```python
from build123d import *

# Parameters (mm, degrees)
F0_R     = 3
F5_DEPTH = 25.501


with BuildPart() as f2:
    # F0 (on Front) → F2 (revolve)
    with BuildSketch(Plane.XZ):
        with BuildLine():
            ThreePointArc((-8, -6), (-15.455298, -3.701711), (-22.32268, 0))
            Line((-22.32268, 0), (-30, 0))
            Line((-30, 0), (-30, -32))
            ThreePointArc((-30, -32), (-22.5, -39.5), (-15, -32))
            Line((-15, -32), (-15, -14))
            Line((-15, -14), (-8, -14))
            Line((-8, -14), (-8, -6))
        make_face()
        with Locations((-22.5, -32)):
            Circle(F0_R, mode=Mode.SUBTRACT)
    revolve(axis=Axis((0, 0, -7), (0, 0, -1)))

    # F4 (on offset) → F5 (cut, through all)
    with BuildSketch(Plane.XY.offset(-14)):
        with BuildLine():
            Line((-2.886751, 5), (10.460072, 28.117377))
            ThreePointArc((10.460072, 28.117377), (-15, 25.980762), (-29.580399, 5))
            Line((-29.580399, 5), (-2.886751, 5))
        make_face()
        with BuildLine():
            ThreePointArc((19.120326, -23.117377), (27.14415, -12.774784), (30, 0))
            ThreePointArc((30, 0), (27.14415, 12.774784), (19.120326, 23.117377))
            Line((19.120326, 23.117377), (5.773503, 0))
            Line((5.773503, 0), (19.120326, -23.117377))
        make_face()
        with BuildLine():
            ThreePointArc((-29.580399, -5), (-15, -25.980762), (10.460072, -28.117377))
            Line((10.460072, -28.117377), (-2.886751, -5))
            Line((-2.886751, -5), (-29.580399, -5))
        make_face()
    extrude(amount=-F5_DEPTH, mode=Mode.SUBTRACT)


solid = f2.part
```
Design review of the part built by this model. Coordinates are the model's own, in mm. A direction names the side the tool comes from. Round coordinates to 2 decimals unless told otherwise and drop trailing zeros. Write each loop counter-clockwise with the first axis right and the second up, starting at its lowest first coordinate (ties: lowest second). Pieces come first, ordered by that corner, then holes. Notation, with made-up numbers: (27.5, 2.25) -> (48.5, 2.25) arc R24 ccw to (48.5, 41.25) -> close; hole circle Ø8 at (-22, 22.25). An arc over 180 degrees is marked (long way). Answer in a Markdown table with one row per item.
Q1. Take a section at C-C, the plane y = -2. Count the separate pieces of the cut face and the enclosed holes in it, then the cut area to 3 significant figures.
The answers:
| item | result |
|---|---|
| separate pieces | 2 |
| enclosed holes | 1 |
| area | 850 mm² |
Q2. Clearance check with flat-ended pins moving along their axes: pin 1 Ø4 at (x, z) = (7.5, -18.5) entering from +Y; pin 2 Ø3 at (x, y) = (14, 12.5) entering from +Z; pin 3 Ø1 at (y, z) = (-17.5, -29.5) entering from +X; pin 4 Ø6 at (x, z) = (-1, -25.5) entering from -Y. State where each tip first meets the part, or that it passes through.
The answers:
| item | result |
|---|---|
| pin 1 | y = 26.45 |
| pin 2 | z = -1.29 |
| pin 3 | x = 16.17 |
| pin 4 | through |
Q3. Draft analysis for pull direction Y (two halves, no side actions). For faces 1 (the face through (6.546, 21.339, -26.573)), 2 (the face through (6.503, -29.287, -5.557)), 3 (the face through (-6, -6, -14)), 4 (the face through (-22, -5, -27)), state which applies: +Y half, -Y half, draft (parallel to the pull), parting line (faces both ways), or undercut.
The answers:
| item | result |
|---|---|
| face 1 | +Y half |
| face 2 | parting line |
| face 3 | undercut |
| face 4 | -Y half |
Q4. Take a section at A-A, the plane z = -22.5. State the section outline as (x, y) points.
The answers:
| item | result |
|---|---|
| outline | (-29.58, -5) -> (-14.14, -5) arc R15 cw to (-14.14, 5) -> (-29.58, 5) arc R30 ccw to start; (2.74, -14.75) -> (10.46, -28.12) arc R30 ccw to (19.12, -23.12) -> (11.4, -9.75) arc R15 cw to start; (2.74, 14.75) arc R15 cw to (11.4, 9.75) -> (19.12, 23.12) arc R30 ccw to (10.46, 28.12) -> close |
Q5. To check wall thickness, follow L1, parallel to Y at x = 0, z = -8; L2, parallel to Z at x = -18, y = 14.5; L3, parallel to X at y = 0.5, z = -31. State the ranges of each line that lie inside material, in increasing order. Write a range as [from, to].
The answers:
| item | result |
|---|---|
| L1 | [-30, -8], [8, 30] |
| L2 | [-14, 0] |
| L3 | [-30, -25.32], [-19.67, -14.99] |
Q6. Take a section at D-D, the plane z = -8.5. State the section outline as (x, y) points.
The answers:
| item | result |
|---|---|
| outline | circle Ø60 at (0, 0); hole circle Ø16 at (0, 0) |
Q7. For faces 5 (the face through (-22, 5, -27)), 6 (the face through (6.655, -21.526, -26.573)), 7 (the face through (15.3, 16.5, -26.6)), 8 (the face through (7.438, 13.026, -22.874)), list the 3-axis set-ups (+Z, -Z, +X, -X, +Y, -Y) from which the entire face can be reached by the end or side of a thin tool; tool diameter is ignored.
The answers:
| item | result |
|---|---|
| face 5 | -Z, +X, -X, +Y |
| face 6 | -Z, -X, -Y |
| face 7 | -Z, +X |
| face 8 | -Z, -X |
Q8. Take a section at B-B, the plane z = -30.5. State the section outline as (x, y) points, then the cut area to 3 significant figures.
The answers:
| item | result |
|---|---|
| outline | (-29.58, -5) -> (-24.59, -5) arc R25.1 cw to (-24.59, 5) -> (-29.58, 5) arc R30 ccw to start; (-19.26, -5) -> (-14.14, -5) arc R15 cw to (-14.14, 5) -> (-19.26, 5) arc R19.9 ccw to start; (2.74, -14.75) -> (5.3, -19.18) arc R19.9 ccw to (13.96, -14.18) -> (11.4, -9.75) arc R15 cw to start; (2.74, 14.75) arc R15 cw to (11.4, 9.75) -> (13.96, 14.18) arc R19.9 ccw to (5.3, 19.18) -> close; (7.97, -23.8) -> (10.46, -28.12) arc R30 ccw to (19.12, -23.12) -> (16.63, -18.8) arc R25.1 cw to start; (7.97, 23.8) arc R25.1 cw to (16.63, 18.8) -> (19.12, 23.12) arc R30 ccw to (10.46, 28.12) -> close |
| area | 297 mm² |
